from build123d import *

# Parameters (mm, degrees)
SALIENTE_EXTRUIR1_DEPTH = 3


with BuildPart() as part:
    # Croquis2 → Saliente-Extruir1 (new body)
    with BuildSketch(Plane.XY):
        Polygon((-32.5, 0), (-25.6, 0), (-25.6, 3), (-13, 3), (-13, 0), (-6.3, 0), (-6.3, 3), (6.3, 3), (6.3, 0), (13, 0), (13, 3), (25.6, 3), (25.6, 0), (32.5, 0), (32.5, -158), (25.6, -158), (25.6, -161), (13, -161), (13, -158), (6.3, -158), (6.3, -161), (-6.3, -161), (-6.3, -158), (-13, -158), (-13, -161), (-25.6, -161), (-25.6, -158), (-32.5, -158), align=None)
        Polygon((-13.175, -7.03), (-25.475, -19.33), (-25.475, -7.03), align=None, mode=Mode.SUBTRACT)
        Polygon((13.175, -7.03), (25.475, -7.03), (25.475, -19.33), align=None, mode=Mode.SUBTRACT)
        Polygon((13.175, -79), (25.475, -66.7), (25.475, -91.3), align=None, mode=Mode.SUBTRACT)
        Polygon((13.175, -150.97), (25.475, -138.67), (25.475, -150.97), align=None, mode=Mode.SUBTRACT)
        Polygon((-13.175, -79), (-25.475, -66.7), (-25.475, -91.3), align=None, mode=Mode.SUBTRACT)
        Polygon((13.175, -43.015), (25.475, -55.315), (25.475, -30.715), align=None, mode=Mode.SUBTRACT)
        Polygon((-13.175, -43.015), (-25.475, -30.715), (-25.475, -55.315), align=None, mode=Mode.SUBTRACT)
        Polygon((0, -48.7075), (-12.3, -61.0075), (0, -73.3075), (12.3, -61.0075), align=None, mode=Mode.SUBTRACT)
        Polygon((0, -12.7225), (12.3, -25.0225), (0, -37.3225), (-12.3, -25.0225), align=None, mode=Mode.SUBTRACT)
        Polygon((-13.175, -150.97), (-25.475, -150.97), (-25.475, -138.67), align=None, mode=Mode.SUBTRACT)
        Polygon((-13.175, -114.985), (-25.475, -127.285), (-25.475, -102.685), align=None, mode=Mode.SUBTRACT)
        Polygon((-12.3, -132.9775), (0, -145.2775), (12.3, -132.9775), (0, -120.6775), align=None, mode=Mode.SUBTRACT)
        Polygon((13.175, -114.985), (25.475, -127.285), (25.475, -102.685), align=None, mode=Mode.SUBTRACT)
        Polygon((0, -84.6925), (12.3, -96.9925), (0, -109.2925), (-12.3, -96.9925), align=None, mode=Mode.SUBTRACT)
    extrude(amount=SALIENTE_EXTRUIR1_DEPTH)


solid = part.part
Here's how the part is built. I have some questions about the finished solid (model axes, mm). A direction names the side the tool comes from. Coordinates: 2 decimals unless noted, no trailing zeros. Order: outer loops, then holes, each group sorted by start corner. A loop starts at its lowest first (then second) coordinate and runs counter-clockwise, first axis right, second up. Notation, with made-up numbers: M 2,-13.5 L 13,-13.5 A14 ccw 13,9.5 Z; hole C 69,69.25 d7. An arc over 180 degrees is marked long. Answer as CSV lines item,"result". Start each with the question number.
1. I want a section at A-A, the plane x = 3.5. Write out the boundary of the cut face in (y, z).
2. I want a section at C-C, the plane x = 16.5. Write out the boundary of the cut face in (y, z) (3 decimals).
3. I want a section at B-B, the plane y = -62.5. Write out the boundary of the cut face in (x, z), and give its area (3 significant figures).
4. On a 3-axis mill with a long thin cutter (end or side, diameter ignored), from which of +Z, -Z, +X, -X, +Y, -Y can I reach the whole of each face in a straight line? I mean faces 1 (the flat face through (-6.3, -160, 1)), 2 (the flat face through (-6.3, 1, 1)), 3 (the flat face through (19.411, -85.236, 1.479)). Say none if no direction works.
5. I need wall thicknesses on line 1 (Y direction, x = -10, z = 1); line 2 (X direction, y = -50, z = 1.1) (1 decimal); line 3 (Y direction, x = -5.5, z = 0.45). Which ranges of each line are inside material? Lowest first, please. Write a range as [from, to].
6. We'd pull the mould along Y, two halves only. Please class faces 4 (the flat face through (6.3, 2, 1)), 5 (the flat face through (-10, 0, 1)), 6 (the flat face through (6.236, -31.086, 1.479)): released by +Y, released by -Y, zero draft, split by the parting line, or undercut.
7. For pin 1 (1.5 mm diameter, centred on y = -159, z = 1.5, fed in from -X); pin 2 (1 mm diameter, centred on x = -21.5, y = -99.5, fed in from -Z); pin 3 (1.5 mm diameter, centred on y = -159.5, z = 1.5, fed in from +X); pin 4 (1.5 mm diameter, centred on x = 9, z = 1.5, fed in from -Y), each with a flat end and sliding along its axis, tell me the tip position at first contact or that it passes through.
8. I want a section at D-D, the plane y = -125. Write out the boundary of the cut face in (x, z) (1 decimal), and give its area (3 significant figures).
Recorded:
1,outline,"M -161,0 L -141.78,0 L -141.78,3 L -161,3 Z; M -124.18,0 L -105.79,0 L -105.79,3 L -124.18,3 Z; M -88.19,0 L -69.81,0 L -69.81,3 L -88.19,3 Z; M -52.21,0 L -33.82,0 L -33.82,3 L -52.21,3 Z; M -16.22,0 L 3,0 L 3,3 L -16.22,3 Z"
2,outline,"M -161,0 L -150.97,0 L -150.97,3 L -161,3 Z; M -147.645,0 L -118.31,0 L -118.31,3 L -147.645,3 Z; M -111.66,0 L -82.325,0 L -82.325,3 L -111.66,3 Z; M -75.675,0 L -46.34,0 L -46.34,3 L -75.675,3 Z; M -39.69,0 L -10.355,0 L -10.355,3 L -39.69,3 Z; M -7.03,0 L 3,0 L 3,3 L -7.03,3 Z"
3,outline,"M -32.5,0 L -10.81,0 L -10.81,3 L -32.5,3 Z; M 10.81,0 L 32.5,0 L 32.5,3 L 10.81,3 Z"
3,area,"130 mm2"
4,face 1,"+Z, -Z, -Y"
4,face 2,"+Z, -Z, +Y"
4,face 3,"+Z, -Z"
5,line 1,"y = [-158, -135.28], [-130.68, -99.29], [-94.69, -63.31], [-58.71, -27.32], [-22.72, 0]"
5,line 2,"x = [-32.5, -25.5], [-20.2, -1.3], [1.3, 20.2], [25.5, 32.5]"
5,line 3,"y = [-161, -139.78], [-126.18, -103.79], [-90.19, -67.81], [-54.21, -31.82], [-18.22, 3]"
6,face 4,"zero draft"
6,face 5,"released by +Y"
6,face 6,"undercut"
7,pin 1,"stops at x = -25.6"
7,pin 2,"stops at z = 0"
7,pin 3,"stops at x = 25.6"
7,pin 4,"stops at y = -158"
8,outline,"M -32.5,0 L -25.5,0 L -25.5,3 L -32.5,3 Z; M -23.2,0 L -4.3,0 L -4.3,3 L -23.2,3 Z; M 4.3,0 L 23.2,0 L 23.2,3 L 4.3,3 Z; M 25.5,0 L 32.5,0 L 32.5,3 L 25.5,3 Z"
8,area,"155 mm2"
